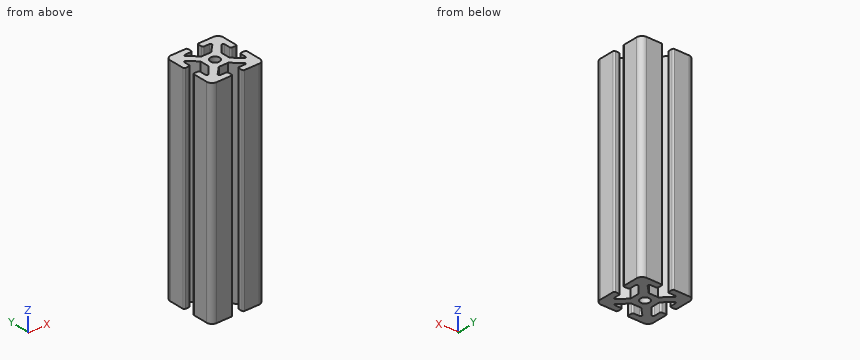
from build123d import *

# Parameters (mm, degrees)
SKETCH2_R           = 3.492543695
BOSS_EXTRUDE1_DEPTH = 160


with BuildPart() as part:
    # Sketch2 → Boss-Extrude1 (new body)
    with BuildSketch(Plane.XY):
        with BuildLine():
            Line((19.48831917, 27.684671829), (23.749889801, 27.684671829))
            Line((23.749889801, 27.684671829), (29.699681879, 33.624984685))
            ThreePointArc((29.699681879, 33.624984685), (29.917171057, 34.714970099), (28.993139054, 35.332654972))
            Line((28.993139054, 35.332654972), (24.845630957, 35.332654972))
            ThreePointArc((24.845630957, 35.332654972), (24.138524175, 35.625548191), (23.845630957, 36.332654972))
            Line((23.845630957, 36.332654972), (23.845630957, 39))
            ThreePointArc((23.845630957, 39), (24.138524175, 39.707106781), (24.845630957, 40))
            Line((24.845630957, 40), (36, 40))
            ThreePointArc((36, 40), (38.828427125, 38.828427125), (40, 36))
            Line((40, 36), (40, 24.961087436))
            ThreePointArc((40, 24.961087436), (39.707106781, 24.253980655), (39, 23.961087436))
            Line((39, 23.961087436), (36.388269628, 23.961087436))
            ThreePointArc((36.388269628, 23.961087436), (35.681162846, 24.253980655), (35.388269628, 24.961087436))
            Line((35.388269628, 24.961087436), (35.388269628, 29.408620307))
            ThreePointArc((35.388269628, 29.408620307), (34.744223919, 30.343123673), (33.641676542, 30.073901274))
            Line((33.641676542, 30.073901274), (27.684671829, 23.388818206))
            Line((27.684671829, 23.388818206), (27.684671829, 20.51168083))
            Line((27.684671829, 20.51168083), (27.684671829, 16.250110199))
            Line((27.684671829, 16.250110199), (33.624984685, 10.300318121))
            ThreePointArc((33.624984685, 10.300318121), (34.714970099, 10.082828943), (35.332654972, 11.006860946))
            Line((35.332654972, 11.006860946), (35.332654972, 15.154369043))
            ThreePointArc((35.332654972, 15.154369043), (35.625548191, 15.861475825), (36.332654972, 16.154369043))
            Line((36.332654972, 16.154369043), (39, 16.154369043))
            ThreePointArc((39, 16.154369043), (39.707106781, 15.861475825), (40, 15.154369043))
            Line((40, 15.154369043), (40, 4))
            ThreePointArc((40, 4), (38.828427125, 1.171572875), (36, 0))
            Line((36, 0), (24.961087436, 0))
            ThreePointArc((24.961087436, 0), (24.253980655, 0.292893219), (23.961087436, 1))
            Line((23.961087436, 1), (23.961087436, 3.611730372))
            ThreePointArc((23.961087436, 3.611730372), (24.253980655, 4.318837154), (24.961087436, 4.611730372))
            Line((24.961087436, 4.611730372), (29.408620307, 4.611730372))
            ThreePointArc((29.408620307, 4.611730372), (30.343123673, 5.255776081), (30.073901274, 6.358323458))
            Line((30.073901274, 6.358323458), (23.388818206, 12.315328171))
            Line((23.388818206, 12.315328171), (20.51168083, 12.315328171))
            Line((20.51168083, 12.315328171), (16.250110199, 12.315328171))
            Line((16.250110199, 12.315328171), (10.300318121, 6.375015315))
            ThreePointArc((10.300318121, 6.375015315), (10.082828943, 5.285029901), (11.006860946, 4.667345028))
            Line((11.006860946, 4.667345028), (15.154369043, 4.667345028))
            ThreePointArc((15.154369043, 4.667345028), (15.861475825, 4.374451809), (16.154369043, 3.667345028))
            Line((16.154369043, 3.667345028), (16.154369043, 1))
            ThreePointArc((16.154369043, 1), (15.861475825, 0.292893219), (15.154369043, 0))
            Line((15.154369043, 0), (4, 0))
            ThreePointArc((4, 0), (1.171572875, 1.171572875), (0, 4))
            Line((0, 4), (0, 15.038912564))
            ThreePointArc((0, 15.038912564), (0.292893219, 15.746019345), (1, 16.038912564))
            Line((1, 16.038912564), (3.611730372, 16.038912564))
            ThreePointArc((3.611730372, 16.038912564), (4.318837154, 15.746019345), (4.611730372, 15.038912564))
            Line((4.611730372, 15.038912564), (4.611730372, 10.591379693))
            ThreePointArc((4.611730372, 10.591379693), (5.255776081, 9.656876327), (6.358323458, 9.926098726))
            Line((6.358323458, 9.926098726), (12.315328171, 16.611181794))
            Line((12.315328171, 16.611181794), (12.315328171, 19.48831917))
            Line((12.315328171, 19.48831917), (12.315328171, 23.749889801))
            Line((12.315328171, 23.749889801), (6.375015315, 29.699681879))
            ThreePointArc((6.375015315, 29.699681879), (5.285029901, 29.917171057), (4.667345028, 28.993139054))
            Line((4.667345028, 28.993139054), (4.667345028, 24.845630957))
            ThreePointArc((4.667345028, 24.845630957), (4.374451809, 24.138524175), (3.667345028, 23.845630957))
            Line((3.667345028, 23.845630957), (1, 23.845630957))
            ThreePointArc((1, 23.845630957), (0.292893219, 24.138524175), (0, 24.845630957))
            Line((0, 24.845630957), (0, 36))
            ThreePointArc((0, 36), (1.171572875, 38.828427125), (4, 40))
            Line((4, 40), (15.038912564, 40))
            ThreePointArc((15.038912564, 40), (15.746019345, 39.707106781), (16.038912564, 39))
            Line((16.038912564, 39), (16.038912564, 36.388269628))
            ThreePointArc((16.038912564, 36.388269628), (15.746019345, 35.681162846), (15.038912564, 35.388269628))
            Line((15.038912564, 35.388269628), (10.591379693, 35.388269628))
            ThreePointArc((10.591379693, 35.388269628), (9.656876327, 34.744223919), (9.926098726, 33.641676542))
            Line((9.926098726, 33.641676542), (16.611181794, 27.684671829))
            Line((16.611181794, 27.684671829), (19.48831917, 27.684671829))
        make_face()
        with Locations((20, 20)):
            Circle(SKETCH2_R, mode=Mode.SUBTRACT)
    extrude(amount=BOSS_EXTRUDE1_DEPTH)


solid = part.part
Build history of the part. All positions in model axes, mm. Give positions to 0.01 mm unless a question says otherwise; leave off trailing zeros. Order: outer loops, then holes, each group sorted by start corner. A loop starts at its lowest first (then second) coordinate and runs counter-clockwise, first axis right, second up. Notation, with made-up numbers: M 52.5,-5.5 L 72.5,-5.5 A26 ccw 72.5,10.5 Z; hole C 21.25,15.5 d1. An arc over 180 degrees is marked long. Put each result on its own line as item: value.
Item 1: Cut at A-A on y = 20. Write the cut outline in (x, z), then the cut area to 3 significant figures.
Results are:
outline: M 12.32,0 L 16.51,0 L 16.51,160 L 12.32,160 Z; M 23.49,0 L 27.68,0 L 27.68,160 L 23.49,160 Z
area: 1,340 mm2
Item 2: Wall check: probe 1 along Y at (x, z) = (27, 134.5); probe 2 along X at (y, z) = (36.5, 120.5); probe 3 along Y at (x, z) = (20, 65). Give the ranges that are in metal, low to high.
Results are:
probe 1: 0 to 4.61, 9.1 to 30.93, 35.33 to 40
probe 2: 0.03 to 16.04, 23.85 to 39.97
probe 3: 12.32 to 16.51, 23.49 to 27.68
Item 3: Drop flat-ended pins along their axis: pin 1 Ø0.8 at (y, z) = (38.5, 100.5) entering from +X; pin 2 Ø6.5 at (x, y) = (20, 20) entering from -Z; pin 3 Ø1.3 at (x, z) = (1.5, 82.5) entering from +Y; pin 4 Ø2 at (x, z) = (20.5, 54.5) entering from -Y. Give the stop position or say it passes through.
Results are:
pin 1: x = 39.4
pin 2: through
pin 3: y = 39.55
pin 4: y = 12.32
